from build123d import *

# Parameters (mm, degrees)
SKETCH_1_W          = 24
SKETCH_1_H          = 36
EXTRUDE_1_DEPTH     = 2
FILLET_1_R          = 2
SKETCH_4_R          = 2.05
CUT_EXTRUDE_1_DEPTH = 1
SKETCH_9_R          = 1
CUT_EXTRUDE_3_DEPTH = 1
CUT_EXTRUDE_4_REACH = 146.484
SKETCH_10_R         = 0.5


with BuildPart() as part:
    # 草图1 → 凸台-拉伸1 (new body)
    with BuildSketch(Plane.XY):
        with Locations((-109.790086771, 59.72858385)):
            Rectangle(SKETCH_1_W, SKETCH_1_H)
    extrude(amount=EXTRUDE_1_DEPTH)

    # 圆角1
    fillet_1_edges = [part.edges().sort_by_distance(p)[0] for p in [
        (-121.790086771, 59.72858385, 2),
        (-109.790086771, 41.72858385, 2),
        (-97.790086771, 59.72858385, 2),
        (-97.790086771, 41.72858385, 1),
        (-121.790086771, 41.72858385, 1),
        (-121.790086771, 77.72858385, 1),
        (-97.790086771, 77.72858385, 1),
        (-109.790086771, 77.72858385, 2),
    ]]
    fillet(fillet_1_edges, radius=FILLET_1_R - 0.0001)  # a hair under: the kernel refuses the full size

    # 草图4 → 切除-拉伸1 (cut)
    with BuildSketch(Plane(origin=(0, 0, 0), x_dir=(-1, 0, 0), z_dir=(0, 0, -1))):
        with Locations((117.950086771, 65.97858385)):
            Circle(SKETCH_4_R)
    extrude(amount=-CUT_EXTRUDE_1_DEPTH, mode=Mode.SUBTRACT)

    # 草图9 → 切除-拉伸3 (cut)
    with BuildSketch(Plane.XY.offset(2)):
        with Locations((-100.790086771, 74.72858385)):
            Circle(SKETCH_9_R)
        with Locations((-100.790086771, 44.72858385)):
            Circle(SKETCH_9_R)
        with Locations((-118.790086771, 44.72858385)):
            Circle(SKETCH_9_R)
        with Locations((-118.790086771, 74.72858385)):
            Circle(SKETCH_9_R)
    extrude(amount=-CUT_EXTRUDE_3_DEPTH, mode=Mode.SUBTRACT)

    # 草图10 → 切除-拉伸4 (cut, up to next)
    with BuildSketch(Plane.XY.offset(1), mode=Mode.PRIVATE) as cut_extrude_4_sk1:
        with Locations((-118.790086771, 44.72858385)):
            Circle(SKETCH_10_R)
    cut_extrude_4_tool1 = extrude(cut_extrude_4_sk1.sketch, amount=-CUT_EXTRUDE_4_REACH, mode=Mode.PRIVATE) & part.part
    # 草图10 → 切除-拉伸4 (cut, up to next)
    with BuildSketch(Plane.XY.offset(1), mode=Mode.PRIVATE) as cut_extrude_4_sk2:
        with Locations((-100.790086771, 44.72858385)):
            Circle(SKETCH_10_R)
    cut_extrude_4_tool2 = extrude(cut_extrude_4_sk2.sketch, amount=-CUT_EXTRUDE_4_REACH, mode=Mode.PRIVATE) & part.part
    # 草图10 → 切除-拉伸4 (cut, up to next)
    with BuildSketch(Plane.XY.offset(1), mode=Mode.PRIVATE) as cut_extrude_4_sk3:
        with Locations((-100.790086771, 74.72858385)):
            Circle(SKETCH_10_R)
    cut_extrude_4_tool3 = extrude(cut_extrude_4_sk3.sketch, amount=-CUT_EXTRUDE_4_REACH, mode=Mode.PRIVATE) & part.part
    # 草图10 → 切除-拉伸4 (cut, up to next)
    with BuildSketch(Plane.XY.offset(1), mode=Mode.PRIVATE) as cut_extrude_4_sk4:
        with Locations((-118.790086771, 74.72858385)):
            Circle(SKETCH_10_R)
    cut_extrude_4_tool4 = extrude(cut_extrude_4_sk4.sketch, amount=-CUT_EXTRUDE_4_REACH, mode=Mode.PRIVATE) & part.part
    add(cut_extrude_4_tool1.solids().sort_by_distance((-118.790087, 44.728584, 1))[0], mode=Mode.SUBTRACT)
    add(cut_extrude_4_tool2.solids().sort_by_distance((-100.790087, 44.728584, 1))[0], mode=Mode.SUBTRACT)
    add(cut_extrude_4_tool3.solids().sort_by_distance((-100.790087, 74.728584, 1))[0], mode=Mode.SUBTRACT)
    add(cut_extrude_4_tool4.solids().sort_by_distance((-118.790087, 74.728584, 1))[0], mode=Mode.SUBTRACT)


solid = part.part
CAD build for the part. Positions are in the model's coordinates, mm. A direction names the side the tool comes from. Round coordinates to 2 decimals unless told otherwise and drop trailing zeros. Write each loop counter-clockwise with the first axis right and the second up, starting at its lowest first coordinate (ties: lowest second). Pieces come first, ordered by that corner, then holes.
(1) Drop flat-ended pins along their axis: P1, Ø2, axis at x = -101, y = 45, coming from the +Z side; P2, Ø0.6, axis at x = -119, y = 75, coming from the +Z side. Give the stop position or say it passes through.
(2) Probe line 1 along Y through (x, z) = (-100.75, 0.5); line 2 along Y through (x, z) = (-106.75, 0.4); line 3 along X through (y, z) = (58, 0.8). List the from-to ranges inside material, lowest first.
(3) Slice it at A-A, the plane z = 0.6. Write the cut outline in (x, y), and give its area (3 significant figures).
(4) Mould opens along X. For faces 1 (the face through (-98.36, 59.95, 1.4)), 2 (the face through (-100, 75, 1)), 3 (the face through (-109.7, 42.3, 1.4)) say: pulls with the +X half, pulls with the -X half, needs draft (parallel to the pull), parting line crosses it, or undercut.
(5) 3-axis set-ups, long thin cutter, end or side, ignore diameter. For faces 4 (the face through (-118, 66, 1)), 5 (the face through (-100.328, 44.537, 0.507)), 6 (the face through (-117.866, 74.346, 1.507)): which of +Z, -Z, +X, -X, +Y, -Y reach the whole face in a straight line?
From the geometry:
1. P1: stops at z = 2
1. P2: stops at z = 1
2. line 1: y = 41.79 to 44.23, 45.23 to 74.23, 75.23 to 77.67
2. line 2: y = 41.77 to 77.69
2. line 3: x = -121.62 to -97.96
3. outline: (-121.7, 43.73) arc R1.91 ccw to (-119.79, 41.82) - (-99.79, 41.82) arc R1.91 ccw to (-97.88, 43.73) - (-97.88, 75.73) arc R1.91 ccw to (-99.79, 77.64) - (-119.79, 77.64) arc R1.91 ccw to (-121.7, 75.73) - close; hole circle Ø4.1 at (-117.95, 65.98); hole circle Ø1 at (-118.79, 44.73); hole circle Ø1 at (-118.79, 74.73); hole circle Ø1 at (-100.79, 44.73); hole circle Ø1 at (-100.79, 74.73)
3. area: 834 mm2
4. face 1: pulls with the +X half
4. face 2: undercut
4. face 3: needs draft
5. face 4: -Z
5. face 5: +Z, -Z
5. face 6: +Z
